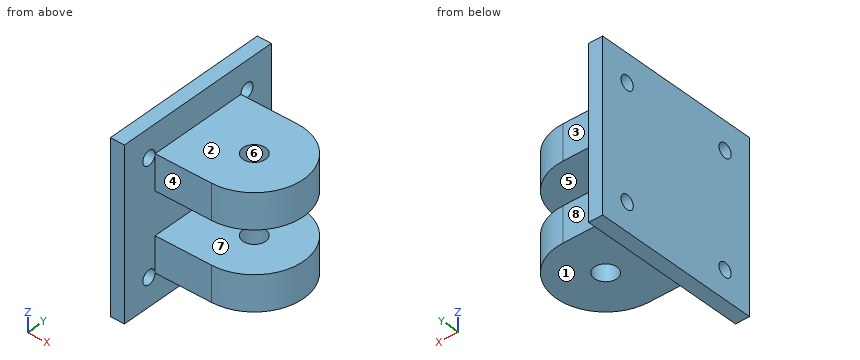
Autodesk Inventor part; units mm, degrees
ref_plane "YZ Plane" through (0, 0, 0) normal (1, 0, 0) x (0, 1, 0)
ref_plane "XZ Plane" through (0, 0, 0) normal (0, 1, 0) x (-1, 0, 0)
ref_plane "XY Plane" through (0, 0, 0) normal (0, 0, 1) x (1, 0, 0)
sketch "Sketch1" plane through (0, 0, 0) normal (1, 0, 0) x (0, 1, 0)
  line L0 (22.5602, 53.0087) -> (-53.6398, 53.0087)
  line L1 (-53.6398, 53.0087) -> (-53.6398, -23.1913)
  line L2 (-53.6398, -23.1913) -> (22.5602, -23.1913)
  line L3 (22.5602, -23.1913) -> (22.5602, 53.0087)
  point P0 (0, 0)
  dimension "d0" = 76.2
  dimension "d1" = 76.2
extrude "Extrusion1" add sketch "Sketch1" along normal blind 6.35
sketch "Sketch2" plane through (6.35, 0, 0) normal (1, 0, 0) x (0, 0, -1)
  line L0 (23.1913, 22.5602) -> (-53.0087, 22.5602)
  line L1 (-53.0087, 22.5602) -> (-53.0087, -53.6398)
  line L2 (23.1913, -53.6398) -> (23.1913, 22.5602)
  line L3 (-53.0087, -53.6398) -> (23.1913, -53.6398)
  point P0 (0, 0)
  point P1 (-40.3087, 9.8602)
  point P2 (10.4913, 9.8602)
  point P3 (-40.3087, -40.9398)
  point P4 (10.4913, -40.9398)
  dimension "d4" = 12.7
  dimension "d5" = 12.7
  dimension "d6" = 12.7
  dimension "d7" = 12.7
  dimension "d8" = 12.7
  dimension "d9" = 12.7
  dimension "d10" = 12.7
  dimension "d11" = 12.7
hole "Hole1" at (6.35, 9.8602, 40.3087) at (6.35, 9.8602, -10.4913) at (6.35, -40.9398, 40.3087) at (6.35, -40.9398, -10.4913) direction (-1, 0, 0) diameter 6.35 end through all
sketch "Sketch3" plane through (0, -53.6398, 53.0087) normal (0, 0, 1) x (1, 0, 0)
  line L0 (6.35, 76.2) -> (6.35, 0)
  line L1 (6.35, 60.325) -> (31.75, 60.325)
  line L2 (31.75, 60.325) -> (31.75, 15.875)
  line L3 (31.75, 15.875) -> (6.35, 15.875)
  line L4 (6.35, 15.875) -> (6.35, 60.325)
  line L5 (0, 76.2) -> (6.35, 76.2)
  arc A0 (31.75, 15.875) -> (31.75, 60.325) centre (31.75, 38.1) ccw
  circle A1 centre (31.75, 38.1) radius 5.08
  point P0 (0, 53.6398)
  point P1 (6.35, 15.875)
  dimension "d19" = 25.4
  dimension "d20" = 44.45
  dimension "d21" = 15.875
  dimension "d22" = 10.16
extrude "Extrusion2" add sketch "Sketch3" against normal blind 76.2 contours L1 L2 A1 L3 L0 | A0 L2 A1
sketch "Sketch4" plane through (6.35, 6.6852, 53.0087) normal (0, 1, 0) x (1, 0, 0)
  line L0 (25.4, 0) -> (0, 0)
  line L1 (0, 0) -> (74.1036, 0)
  line L2 (74.1036, 0) -> (74.1036, 12.7)
  line L3 (74.1036, 12.7) -> (0, 12.7)
  line L4 (0, 12.7) -> (0, 0)
  line L5 (-6.35, 76.2) -> (0, 76.2)
  line L6 (0, 76.2) -> (74.1036, 76.2)
  line L7 (74.1036, 76.2) -> (74.1036, 63.5)
  line L8 (74.1036, 63.5) -> (0, 63.5)
  line L9 (0, 63.5) -> (0, 76.2)
  line L10 (0, 28.575) -> (74.1036, 28.575)
  line L11 (74.1036, 28.575) -> (74.1036, 47.625)
  line L12 (74.1036, 47.625) -> (0, 47.625)
  line L13 (0, 47.625) -> (0, 28.575)
  point P0 (-6.35, 53.0087)
  dimension "d25" = 12.7
  dimension "d26" = 12.7
  dimension "d27" = 19.05
  dimension "d28" = 15.875
extrude "Extrusion3" cut sketch "Sketch4" against normal blind 76.2
properties part number "Undercarriage load"
Can you work these out from the model? Positions are in its coordinate system, mm. Face numbers are marked on the shaded views. A direction names the side the tool comes from. Give positions to 0.01 mm unless a question says otherwise; leave off trailing zeros. Write each loop counter-clockwise with the first axis right and the second up, starting at its lowest first coordinate (ties: lowest second). Pieces come first, ordered by that corner, then holes. Notation, with made-up numbers: (-27, 83) -> (-5, 83) arc R11 ccw to (-5, 89) -> close; hole circle Ø11 at (-7.75, -26.5). An arc over 180 degrees is marked (long way). Answer as a JSON object with one key per item and string values. Group by question number.
Item 1: We'd pull the mould along Y, two halves only. Please class the marked faces 6, 7 and 8: +Y half, -Y half, draft (parallel to the pull), parting line (faces both ways), or undercut.
Item 2: Please list where these lines run through material, in increasing order: line 1 (Z direction, x = 11, y = -28); line 2 (Y direction, x = 31.75, z = -4.5); line 3 (X direction, y = -28.5, z = 9). Write a range as [from, to].
Item 3: Suppose I cut it at A-A (x = 20). Please give me the cut outline in (y, z), plus the area to 3 significant figures.
Item 4: I'm going to push flat-ended pins straight in: P1, Ø5, axis at x = 16, z = -6.5, coming from the -Y side; P2, Ø5, axis at x = 16, z = -6.5, coming from the +Y side; P3, Ø4, axis at y = -40.94, z = 40.31, coming from the -X side; P4, Ø10, axis at y = -0.5, z = 11.5, coming from the +X side. Where does each tip first touch, or does it pass through?
Item 5: Suppose I cut it at D-D (y = -12.5). Please give me the cut outline in (x, z), plus the area to 3 significant figures.
Item 6: Suppose I cut it at B-B (z = -12). Please give me the cut outline in (x, y), plus the area to 3 significant figures.
Item 7: Suppose I cut it at C-C (x = 35). Please give me the cut outline in (y, z).
Item 8: For the marked faces 1, 2, 3, 4 and 5, which set-ups out of +Z, -Z, +X, -X, +Y, -Y let a thin tool reach every point of the face, with its end or its side?
Findings:
{
 "1": {"face 6": "undercut", "face 7": "draft", "face 8": "+Y half"},
 "2": {"line 1": "z = [-10.49, 5.38], [24.43, 40.31]", "line 2": "y = [-37.76, -20.62], [-10.46, 6.69]", "line 3": "x = [0, 6.35]"},
 "3": {"outline": "(-37.76, -10.49) -> (6.69, -10.49) -> (6.69, 5.38) -> (-37.76, 5.38) -> close; (-37.76, 24.43) -> (6.69, 24.43) -> (6.69, 40.31) -> (-37.76, 40.31) -> close", "area": "1,410 mm²"},
 "4": {"P1": "stops at y = -37.76", "P2": "stops at y = 6.69", "P3": "passes through", "P4": "stops at x = 6.35"},
 "5": {"outline": "(0, -23.19) -> (6.35, -23.19) -> (6.35, -10.49) -> (27.68, -10.49) -> (27.68, 5.38) -> (6.35, 5.38) -> (6.35, 24.43) -> (27.68, 24.43) -> (27.68, 40.31) -> (6.35, 40.31) -> (6.35, 53.01) -> (0, 53.01) -> close; (35.82, -10.49) -> (53.77, -10.49) -> (53.77, 5.38) -> (35.82, 5.38) -> close; (35.82, 24.43) -> (53.77, 24.43) -> (53.77, 40.31) -> (35.82, 40.31) -> close", "area": "1,730 mm²"},
 "6": {"outline": "(0, -53.64) -> (6.35, -53.64) -> (6.35, -43.73) -> (0, -43.73) -> close; (0, -38.15) -> (6.35, -38.15) -> (6.35, 7.07) -> (0, 7.07) -> close; (0, 12.65) -> (6.35, 12.65) -> (6.35, 22.56) -> (0, 22.56) -> close", "area": "413 mm²"},
 "7": {"outline": "(-37.53, -10.49) -> (-19.44, -10.49) -> (-19.44, 5.38) -> (-37.53, 5.38) -> close; (-37.53, 24.43) -> (-19.44, 24.43) -> (-19.44, 40.31) -> (-37.53, 40.31) -> close; (-11.64, -10.49) -> (6.45, -10.49) -> (6.45, 5.38) -> (-11.64, 5.38) -> close; (-11.64, 24.43) -> (6.45, 24.43) -> (6.45, 40.31) -> (-11.64, 40.31) -> close"},
 "8": {"face 1": "-Z, +X, +Y, -Y", "face 2": "+Z, +X, +Y, -Y", "face 3": "+Z, -Z, +X, +Y", "face 4": "+Z, -Z, +X, -Y", "face 5": "+X, +Y, -Y"}
}
